Build history of the part. All positions in model axes, mm. A direction names the side the tool comes from. Round coordinates to 2 decimals unless told otherwise and drop trailing zeros. Write each loop counter-clockwise with the first axis right and the second up, starting at its lowest first coordinate (ties: lowest second). Pieces come first, ordered by that corner, then holes. Notation, with made-up numbers: (30.25, 70) -> (44.25, 70) arc R10 cw to (44.25, 86) -> close; hole circle Ø11 at (-39, 16.5). An arc over 180 degrees is marked (long way). Answer in a Markdown table with one row per item.
```python
from build123d import *

# Parameters (mm, degrees)
SKETCH1_R           = 75
BOSS_EXTRUDE1_DEPTH = 10
CHAMFER1_SIZE       = 8
SHELL1_T            = -3
SKETCH2_R           = 1.75
CUT_EXTRUDE1_DEPTH  = 107.536378763


with BuildPart() as part:
    # Sketch1 → Boss-Extrude1 (new body)
    with BuildSketch(Plane.XY):
        Circle(SKETCH1_R)
    extrude(amount=BOSS_EXTRUDE1_DEPTH)

    # Chamfer1
    chamfer1_edges = [part.edges().sort_by_distance(p)[0] for p in [
        (-75, 0, 0),
    ]]
    chamfer(chamfer1_edges, length=CHAMFER1_SIZE)

    # Shell1
    shell1_openings = [part.faces().sort_by_distance(p)[0] for p in [
        (0, 0, 10),
    ]]
    offset(amount=SHELL1_T, openings=shell1_openings, kind=Kind.INTERSECTION)

    # Sketch2 → Cut-Extrude1 (cut, through all)
    with BuildSketch(Plane(origin=(0, 0, 0), x_dir=(-1, 0, 0), z_dir=(0, 0, -1))):
        with Locations((-50, 15)):
            Circle(SKETCH2_R)
        with Locations((-50, -15)):
            Circle(SKETCH2_R)
        with Locations((-15, -50)):
            Circle(SKETCH2_R)
        with Locations((15, -50)):
            Circle(SKETCH2_R)
        with Locations((50, -15)):
            Circle(SKETCH2_R)
        with Locations((50, 15)):
            Circle(SKETCH2_R)
        with Locations((-15, 50)):
            Circle(SKETCH2_R)
        with Locations((15, 50)):
            Circle(SKETCH2_R)
    extrude(amount=-CUT_EXTRUDE1_DEPTH, mode=Mode.SUBTRACT)


solid = part.part
```
Q1. Saw through at A-A on y = 0. Write the cut outline in (x, z).
A:
| item | result |
|---|---|
| outline | (-75, 8) -> (-67, 0) -> (67, 0) -> (75, 8) -> (75, 10) -> (72, 10) -> (72, 9.24) -> (65.76, 3) -> (-65.76, 3) -> (-72, 9.24) -> (-72, 10) -> (-75, 10) -> close |
Q2. Two-plate mould, pull along X, no slides. Class faces 1 (the conical face through (62.25, -25.81, 0.39)), 2 (the cylindrical face through (-14.62, -51.71, 1.48)), 3 (the flat face through (-1, 1, 0)): released by +X, released by -X, zero draft, split by the parting line, or undercut.
A:
| item | result |
|---|---|
| face 1 | split by the parting line |
| face 2 | undercut |
| face 3 | zero draft |
Q3. Saw through at C-C on x = -50. State how many separate pieces and enclosed holes the cut face has, plus the area to 3 significant figures.
A:
| item | result |
|---|---|
| separate pieces | 3 |
| enclosed holes | 0 |
| area | 339 mm² |
Q4. Which spindle directions (+Z, -Z, +X, -X, +Y, -Y) get a long thin tool onto all of the face, cutting with end or side? Do faces 4 (the cylindrical face through (-14.62, 48.29, 1.48)), 5 (the cylindrical face through (-9.373, 71.387, 9.616)). Say none if no direction does.
A:
| item | result |
|---|---|
| face 4 | +Z, -Z |
| face 5 | +Z |
Q5. Drop flat-ended pins along their axis: P1, Ø3, axis at x = -15, y = 50, coming from the +Z side; P2, Ø5, axis at x = 58, z = 6, coming from the +Y side; P3, Ø5.5, axis at x = -15, y = -50, coming from the +Z side; P4, Ø4, axis at x = 22.5, z = 6.5, coming from the -Y side. Give the stop position or say it passes through.
A:
| item | result |
|---|---|
| P1 | through |
| P2 | y = 49.32 |
| P3 | z = 3 |
| P4 | y = -71.95 |
Q6. Wall check: line 1 (Y direction, x = -50, z = 1.25); line 2 (Y direction, x = 15, z = 1.1); line 3 (Y direction, x = 0, z = 9.4). Give the ranges that are in metal, low to high. Write a range as [from, to].
A:
| item | result |
|---|---|
| line 1 | [-46.45, -16.75], [-13.25, 13.25], [16.75, 46.45] |
| line 2 | [-66.43, -51.75], [-48.25, 48.25], [51.75, 66.43] |
| line 3 | [-75, -72], [72, 75] |
Q7. Saw through at B-B on z = 5. Write the cut outline in (x, y), plus the area to 3 significant figures.
A:
| item | result |
|---|---|
| outline | circle Ø144 at (0, 0); hole circle Ø135.51 at (0, 0) |
| area | 1,860 mm² |
